Geometry: final body of the model. Coordinates: model frame, mm. A direction names the side the tool comes from. Give positions to 0.01 mm unless a question says otherwise; leave off trailing zeros. Order: outer loops, then holes, each group sorted by start corner. A loop starts at its lowest first (then second) coordinate and runs counter-clockwise, first axis right, second up. Notation, with made-up numbers: (53, -4) - (108, -4) arc R10 ccw to (108, 10) - close; hole circle Ø7 at (-21, 13.5). An arc over 180 degrees is marked (long way). One line per item, written item: value.
```python
from build123d import *

# Parameters (mm, degrees)
F0_W     = 18
F0_H     = 10
F1_DEPTH = 20
F1_TAPER = 3
F2_R     = 2.5
F3_DEPTH = 5
F5_R     = 1
F4_R     = 1.5
F6_DEPTH = 25.4


with BuildPart() as f1:
    # F0 (on Top) → F1 (new body)
    with BuildSketch(Plane.XY):
        Rectangle(F0_W, F0_H)
    extrude(amount=F1_DEPTH, taper=F1_TAPER)

    # F2 (on face) → F3 (join)
    with BuildSketch(Plane.XY.offset(20)):
        Circle(F2_R)
    extrude(amount=F3_DEPTH)

    # F5
    f5_edges = [f1.edges().sort_by_distance(p)[0] for p in [
        (8.475922, 4.475922, 10),
        (0, 3.951844, 20),
        (-8.475922, 4.475922, 10),
        (-7.951844, 0, 20),
        (-8.475922, -4.475922, 10),
        (8.475922, -4.475922, 10),
        (0, -3.951844, 20),
        (7.951844, 0, 20),
    ]]
    fillet(f5_edges, radius=F5_R)

    # F4 (on face) → F6 (cut)
    with BuildSketch(Plane(origin=(-8.9753485292, 0, 0.4703780847), x_dir=(0, -1, 0), z_dir=(-0.9986295348, 0, 0.0523359562))):
        with Locations((0, 16.5564233138)):
            Circle(F4_R)
    extrude(amount=-F6_DEPTH, mode=Mode.SUBTRACT)


solid = f1.part
```
1) Material intervals for line 1 along Z through (x, y) = (1, 0.5); line 2 along Z through (x, y) = (6.75, -2.5); line 3 along Z through (x, y) = (3, 1.25), sorted ascending.
Answers below:
line 1: 0 to 15.11, 17.94 to 25
line 2: 0 to 20
line 3: 0 to 15.59, 17.25 to 20
2) Section A-A, the plane y = 0. Return loops of the section in (x, z), then the cut area to 3 significant figures.
Answers below:
outline: (-9, 0) - (9, 0) - (8.23, 14.65) - (-8.19, 15.51) - close; (-8.03, 18.5) - (8.07, 17.66) - (8, 19.05) arc R1 ccw to (7, 20) - (2.5, 20) - (2.5, 25) - (-2.5, 25) - (-2.5, 20) - (-7, 20) arc R1 ccw to (-8, 19.05) - close
area: 315 mm^2
3) Mould query, pull axis Y, two halves, no side actions, for faces 3 (the face through (-8.62, -0.06, 7.28)), 4 (the face through (-8.2, -4.2, 9.7)), 5 (the face through (0.08, 0.195, 18.064)). Classes: released by +Y, released by -Y, zero draft, split by the parting line, or undercut.
Answers below:
face 3: zero draft
face 4: released by -Y
face 5: undercut
4) Set-up query: faces 1 (the face through (7.699, 0.042, 19.718)), 2 (the face through (-0.54, -2.44, 22.46)). Return all of +Z, -Z, +X, -X, +Y, -Y with unobstructed straight access to the full face (end or side cutting, diameter ignored); none if empty.
Answers below:
face 1: +Z, +X, +Y, -Y
face 2: +Z
5) Section B-B, the plane z = 21.75. Return loops of the section in (x, y).
Answers below:
outline: circle Ø5 at (0, 0)
6) First-contact query: pin 1 (1 mm diameter, centred on x = 3.5, y = 1.5, fed in from +Z); pin 2 (8 mm diameter, centred on x = 2.5, z = 18, fed in from +Y); pin 3 (4 mm diameter, centred on x = -0.5, z = 11, fed in from +Y). Flat tips, straight axial feed; report the tip coordinate or a pass-through.
Answers below:
pin 1: z = 20
pin 2: y = 4.27
pin 3: y = 4.53
